```python
from build123d import *

# Parameters (mm, degrees)
F0_W     = 19.97
F0_H     = 19.76
F1_DEPTH = 20.22
F3_DEPTH = 18.76
F2_W     = 14.97
F2_H     = 1.75
F4_DEPTH = 17


with BuildPart() as f1:
    # F0 (on Front) → F1 (new body)
    with BuildSketch(Plane.XZ):
        Rectangle(F0_W, F0_H)
    extrude(amount=F1_DEPTH)

    # F2 (on face) → F3 (cut)
    with BuildSketch(Plane(origin=(0, 0, -9.88), x_dir=(1, 0, 0), z_dir=(0, 0, -1))):
        Polygon((8.985, 1.75), (8.985, 19.22), (-8.985, 19.22), (-8.985, 1.75), (-7.485, 1.75), (7.485, 1.75), align=None)
    extrude(amount=-F3_DEPTH, mode=Mode.SUBTRACT)

    # F2 (on face) → F4 (cut)
    with BuildSketch(Plane(origin=(0, 0, -9.88), x_dir=(1, 0, 0), z_dir=(0, 0, -1))):
        with Locations((0, 0.875)):
            Rectangle(F2_W, F2_H)
        Polygon((8.985, 1.75), (8.985, 19.22), (-8.985, 19.22), (-8.985, 1.75), (-7.485, 1.75), (7.485, 1.75), align=None)
    extrude(amount=-F4_DEPTH, mode=Mode.SUBTRACT)


solid = f1.part
```
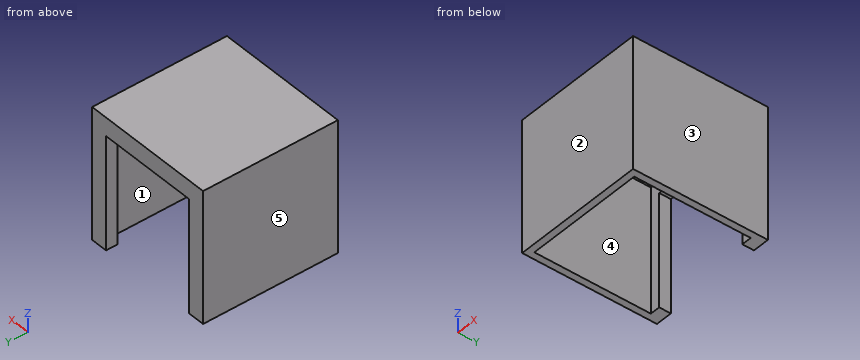
Model file for the job. Use its own axes, mm. Face numbers are marked on the shaded views. A direction names the side the tool comes from. Give positions to 0.01 mm unless a question says otherwise; leave off trailing zeros. Write each loop counter-clockwise with the first axis right and the second up, starting at its lowest first coordinate (ties: lowest second). Pieces come first, ordered by that corner, then holes. Notation, with made-up numbers: M 55.5,1 L 97.5,1 A14 cw 97.5,5 Z; hole C 46.5,-28.75 d1. An arc over 180 degrees is marked long. Use a Markdown table: item, result.
1) Cut at C-C (y = -15.75). List the corners of the cut face in (x, z) (3 decimals).
Responses:
| item | result |
|---|---|
| outline | M -9.985,-9.88 L -8.985,-9.88 L -8.985,8.88 L 8.985,8.88 L 8.985,-9.88 L 9.985,-9.88 L 9.985,9.88 L -9.985,9.88 Z |
2) Pin check, flat tips, straight feed: pin 1 (1 mm diameter, centred on x = -8, y = -7, fed in from -Z); pin 2 (5 mm diameter, centred on x = 2.5, z = 6.5, fed in from +Y); pin 3 (1.4 mm diameter, centred on x = -3, y = -1, fed in from -Z); pin 4 (2 mm diameter, centred on x = -5, z = 4.5, fed in from +Y). Stop position of each tip, or through.
Responses:
| item | result |
|---|---|
| pin 1 | stops at z = 8.88 |
| pin 2 | stops at y = 0 |
| pin 3 | stops at z = 7.12 |
| pin 4 | stops at y = -19.22 |
3) Drill centre lines: line 1 (X direction, y = -19, z = 3.75) (3 decimals); line 2 (Y direction, x = 3.25, z = 8.5); line 3 (Y direction, x = 3.75, z = -6.5). Where is each one in solid material? Low to high. Write a range as from..to.
Responses:
| item | result |
|---|---|
| line 1 | x = -9.985..-8.985, 8.985..9.985 |
| line 2 | y = -20.22..-19.22, -1.75..0 |
| line 3 | y = -20.22..-19.22 |
4) Cut at B-B (z = 2). List the corners of the cut face in (x, y) (3 decimals).
Responses:
| item | result |
|---|---|
| outline | M -9.985,-20.22 L 9.985,-20.22 L 9.985,0 L 7.485,0 L 7.485,-1.75 L 8.985,-1.75 L 8.985,-19.22 L -8.985,-19.22 L -8.985,-1.75 L -7.485,-1.75 L -7.485,0 L -9.985,0 Z |
5) Tool access for the marked faces 4 and 5: list every direction of +Z, -Z, +X, -X, +Y, -Y with a clear straight run to the whole face (end or side of a thin tool).
Responses:
| item | result |
|---|---|
| face 4 | -Z |
| face 5 | +Z, -Z, -X, +Y, -Y |
6) Cut at A-A (x = -8.5). List the corners of the cut face in (y, z), and give its area (3 significant figures).
Responses:
| item | result |
|---|---|
| outline | M -20.22,-9.88 L -19.22,-9.88 L -19.22,8.88 L -1.75,8.88 L -1.75,-9.88 L 0,-9.88 L 0,9.88 L -20.22,9.88 Z |
| area | 71.8 mm2 |
7) Pull direction X, two halves, no side cores. Call the marked faces 1, 2 and 3: +X half, -X half, draft (parallel to the pull), parting line (faces both ways), or undercut.
Responses:
| item | result |
|---|---|
| face 1 | undercut |
| face 2 | draft |
| face 3 | +X half |
